Can you work these out from the model? Positions are in its coordinate system, mm. A direction names the side the tool comes from. Give positions to 0.01 mm unless a question says otherwise; leave off trailing zeros. Loops run counter-clockwise (first coordinate to the right, second up) from the corner with the lowest first, then second, coordinate; pieces in that order, holes last. Notation, with made-up numbers: (85.5, 52.25) - (142.5, 52.25) arc R26 ccw to (142.5, 85.25) - close; hole circle Ø10 at (76.5, 22.25). An arc over 180 degrees is marked (long way). Write item = value, one per line.
from build123d import *

# Parameters (mm, degrees)
SKETCH1_R               = 2.1
BASE_FLANGE1_DEPTH      = 2.5
EDGE_FLANGE1_DEPTH      = 50.5
EDGE_FLANGE2_DEPTH      = 15
EDGE_FLANGE2_START      = 2.5
EDGE_FLANGE2_FLAT_DEPTH = 2.5
EDGE_FLANGE3_DEPTH      = 37.2634
CUT_EXTRUDE1_DEPTH      = 103.451505402
SKETCH18_R              = 8.5
CUT_EXTRUDE2_DEPTH      = 66.845913762
SKETCH19_R              = 2.1
CUT_EXTRUDE3_DEPTH      = 73.336290606


# Sheet-metal steps are written as plain solids
with BuildPart() as part:
    # Sketch1 → Base-Flange1 (new body)
    with BuildSketch(Plane(origin=(0, 0, 0), x_dir=(0, 0, -1), z_dir=(1, 0, 0))):
        Polygon((40.25, 19.5), (44.25, 15.5), (44.25, -11.5), (40.25, -15.5), (-44.25, -15.5), (-44.25, 15.5), (-40.25, 19.5), align=None)
        with Locations((14.25, 7.5)):
            Circle(SKETCH1_R, mode=Mode.SUBTRACT)
        with Locations((14.25, -8.5)):
            Circle(SKETCH1_R, mode=Mode.SUBTRACT)
        with Locations((36.25, 2.5)):
            Circle(SKETCH1_R, mode=Mode.SUBTRACT)
    extrude(amount=-BASE_FLANGE1_DEPTH)

    # Edge-Flange1 section (across the edge) → Edge-Flange1 (add)
    with BuildSketch(Plane(origin=(0, -16.2366, 44.25), x_dir=(0, 1, 0), z_dir=(0, 0, -1))):
        with BuildLine():
            Line((-2.5, 0.7366), (-2.5, 38))
            Line((-2.5, 38), (0, 38))
            Line((0, 38), (0, 0.7366))
            ThreePointArc((0, 0.7366), (0.215745145, 0.215745145), (0.7366, 0))
            Line((0.7366, 0), (0.7366, -2.5))
            ThreePointArc((0.7366, -2.5), (-1.552021808, -1.552021808), (-2.5, 0.7366))
        make_face()
    extrude(amount=EDGE_FLANGE1_DEPTH)

    # Edge-Flange2 bend section (across the edge) → Edge-Flange2 (add)
    with BuildSketch(Plane(origin=(38.7366, -16.2366, 44.25), x_dir=(-1, 0, 0), z_dir=(0, 0, -1))):
        with BuildLine():
            Line((-2.5, 0.7366), (0, 0.7366))
            ThreePointArc((0, 0.7366), (0.215745145, 0.215745145), (0.7366, 0))
            Line((0.7366, 0), (0.7366, -2.5))
            ThreePointArc((0.7366, -2.5), (-1.552021808, -1.552021808), (-2.5, 0.7366))
        make_face()
    extrude(amount=EDGE_FLANGE2_DEPTH)

    # Edge-Flange2 profile (on flange) → Edge-Flange2 flat (add)
    with BuildSketch(Plane(origin=(38.7366, -16.2366, 0), x_dir=(0, 0, -1), z_dir=(1, 0, 0)).offset(EDGE_FLANGE2_START)):
        Polygon((-44.25, 0.7366), (-29.25, 0.7366), (-29.25, 8.5), (-33.25, 12.5), (-40.25, 12.5), (-44.25, 8.5), align=None)
    extrude(amount=-EDGE_FLANGE2_FLAT_DEPTH)

    # Edge-Flange3 section (across the edge) → Edge-Flange3 (add)
    with BuildSketch(Plane(origin=(0.7366, -16.2366, 44.9866), x_dir=(0, 0, -1), z_dir=(1, 0, 0))):
        with BuildLine():
            Line((-2.5, 0.7366), (-2.5, 12.5))
            Line((-2.5, 12.5), (0, 12.5))
            Line((0, 12.5), (0, 0.7366))
            ThreePointArc((0, 0.7366), (0.215745145, 0.215745145), (0.7366, 0))
            Line((0.7366, 0), (0.7366, -2.5))
            ThreePointArc((0.7366, -2.5), (-1.552021808, -1.552021808), (-2.5, 0.7366))
        make_face()
    extrude(amount=EDGE_FLANGE3_DEPTH)

    # Sketch17 → Cut-Extrude1 (cut, through all)
    with BuildSketch(Plane.XY.offset(47.4866)):
        Polygon((0.7366, -7.7366), (4.7366, -3.7366), (0.7366, -3.7366), align=None)
        Polygon((34, -3.7366), (38, -7.7366), (38, -3.7366), align=None)
    extrude(amount=-CUT_EXTRUDE1_DEPTH, mode=Mode.SUBTRACT)

    # Sketch18 → Cut-Extrude2 (cut, through all)
    with BuildSketch(Plane(origin=(0, 0, 0), x_dir=(0, 0, -1), z_dir=(1, 0, 0))):
        with Locations((-24.9866, 8.2634)):
            Circle(SKETCH18_R)
    extrude(amount=-CUT_EXTRUDE2_DEPTH, mode=Mode.SUBTRACT)

    # Sketch19 → Cut-Extrude3 (cut, through all)
    with BuildSketch(Plane(origin=(0, -16.2366, 0), x_dir=(1, 0, 0), z_dir=(0, 1, 0))):
        with Locations(Location((22.5, -26.9866, 0), (0, 0, 180))):
            Circle(SKETCH19_R)
    extrude(amount=-CUT_EXTRUDE3_DEPTH, mode=Mode.SUBTRACT)


solid = part.part
Q1. Imagine slicing it at A-A, the plane z = -14.25. Write out the boundary of the cut face in (x, y).
Output:
outline = (-2.5, -15.5) - (0, -15.5) - (0, -10.6) - (-2.5, -10.6) - close; (-2.5, -6.4) - (0, -6.4) - (0, 5.4) - (-2.5, 5.4) - close; (-2.5, 9.6) - (0, 9.6) - (0, 19.5) - (-2.5, 19.5) - close
Q2. For pin 1 (1 mm diameter, centred on x = 39, y = -11, fed in from -Z); pin 2 (1.2 mm diameter, centred on y = -18, z = 10, fed in from +X); pin 3 (3.5 mm diameter, centred on x = 22.5, z = 26.99, fed in from -Y); pin 4 (3.5 mm diameter, centred on x = 18, y = -17.5, fed in from -Z), each with a flat end and sliding along its axis, tell me the tip position at first contact or that it passes through.
Output:
pin_1 = 29.25
pin_2 = 38
pin_3 = through
pin_4 = -6.25
Q3. We'd pull the mould along Y, two halves only. Please class faces 1 (the cylindrical face through (19.107, -17.814, 46.513)), 2 (the cylindrical face through (-1.232, 5.008, 17.135)), 3 (the cylindrical face through (-1.232, -6.418, -13.977)), 4 (the flat face through (18, -17, -6.25)): released by +Y, released by -Y, zero draft, split by the parting line, or undercut.
Output:
face_1 = released by -Y
face_2 = undercut
face_3 = undercut
face_4 = zero draft
Q4. I need wall thicknesses on L1, parallel to Y at x = -0.6, z = -14.25; L2, parallel to Z at x = -1, y = 2; L3, parallel to X at y = -0.5, z = 11. Which ranges of each line are inside material? Lowest first, please.
Output:
L1 = -15.5 to -10.6, -6.4 to 5.4, 9.6 to 19.5
L2 = -44.25 to -38.29, -34.21 to 19.24, 30.73 to 44.25
L3 = -2.5 to 0
Q5. Imagine slicing it at B-B, the plane x = 22.5. Write out the boundary of the cut face in (y, z), then the cut area to 3 significant figures.
Output:
outline = (-18.74, -6.25) - (-16.24, -6.25) - (-16.24, 24.89) - (-18.74, 24.89) - close; (-18.74, 29.09) - (-16.24, 29.09) - (-16.24, 44.25) arc R0.74 cw to (-15.5, 44.99) - (-3.74, 44.99) - (-3.74, 47.49) - (-15.5, 47.49) arc R3.24 ccw to (-18.74, 44.25) - close
area = 153 mm2
Q6. Which directions (+Z, -Z, +X, -X, +Y, -Y) give clear straight access to the entire face, cutting with the end or side of a thin tool? Please do faces 5 (the flat face through (40, -13, 44.25)), 6 (the flat face through (40, -13, 29.25)), 7 (the flat face through (40.004, -5.765, 31.222)), 8 (the flat face through (0.737, -13, 46)).
Output:
face_5 = +Z, +X, +Y, -Y
face_6 = -Z, +X, +Y, -Y
face_7 = -Z, +X, +Y
face_8 = +Z, -X, +Y, -Y
Q7. Imagine slicing it at C-C, the plane y = -13.5. Write out the boundary of the cut face in (x, z), then the cut area to 3 significant figures.
Output:
outline = (-2.5, -42.25) - (0, -42.25) - (0, 44.25) - (-2.5, 44.25) - close; (0.74, 44.99) - (38, 44.99) - (38, 47.49) - (0.74, 47.49) - close; (38.74, 29.25) - (41.24, 29.25) - (41.24, 44.25) - (38.74, 44.25) - close
area = 347 mm2
Q8. Imagine slicing it at D-D, the plane z = -36.25. Write out the boundary of the cut face in (x, y).
Output:
outline = (-2.5, -15.5) - (0, -15.5) - (0, 0.4) - (-2.5, 0.4) - close; (-2.5, 4.6) - (0, 4.6) - (0, 19.5) - (-2.5, 19.5) - close
